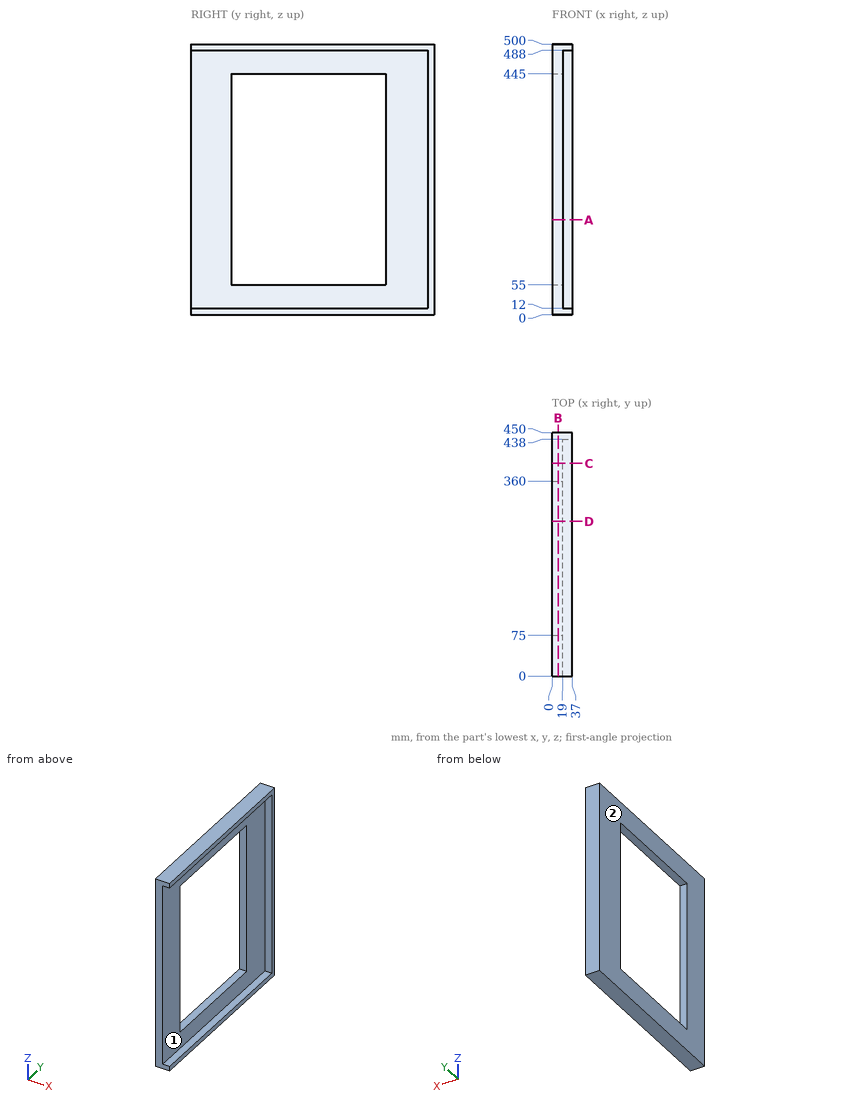
Job drawing, mm, ordinate dimensions from the low corner. One solid piece. Round coordinates to 2 decimals unless told otherwise and drop trailing zeros. Loops run counter-clockwise (first coordinate to the right, second up) from the corner with the lowest first, then second, coordinate; pieces in that order, holes last.
Item 1: Drill centre lines: line 1 (Z direction, x = 18, y = 330); line 2 (Z direction, x = 31.5, y = 383.5); line 3 (Y direction, x = 11.5, z = 184.5). Where is each one in solid material? Low to high.
Item 2: Mould opens along Z. For the marked faces 1 and 2 say: +Z half, -Z half, draft (parallel to the pull), parting line (faces both ways), or undercut.
Item 3: Cut at B-B, the plane x = 11. Give the cut face in (y, z).
Item 4: Cut at C-C, the plane y = 393. Give the cut face in (x, z), then the cut area to 3 significant figures.
Item 5: Cut at D-D, the plane y = 286. Give the cut face in (x, z).
Item 6: Cut at A-A, the plane z = 175. Give the cut face in (x, y), then the cut area to 3 significant figures.
A:
1. line 1: z = 0 to 55, 445 to 500
1. line 2: z = 0 to 12, 488 to 500
1. line 3: y = 0 to 75, 360 to 450
2. face 1: undercut
2. face 2: draft
3. outline: (0, 0) - (450, 0) - (450, 500) - (0, 500) - close; hole (75, 55) - (360, 55) - (360, 445) - (75, 445) - close
4. outline: (0, 0) - (37, 0) - (37, 12) - (19, 12) - (19, 488) - (37, 488) - (37, 500) - (0, 500) - close
4. area: 9,930 mm2
5. outline: (0, 0) - (37, 0) - (37, 12) - (19, 12) - (19, 55) - (0, 55) - close; (0, 445) - (19, 445) - (19, 488) - (37, 488) - (37, 500) - (0, 500) - close
6. outline: (0, 0) - (19, 0) - (19, 75) - (0, 75) - close; (0, 360) - (19, 360) - (19, 438) - (37, 438) - (37, 450) - (0, 450) - close
6. area: 3,350 mm2
